Here's how the part is built. I have some questions about the finished solid (model axes, mm). Give positions to 0.01 mm unless a question says otherwise; leave off trailing zeros. Write each loop counter-clockwise with the first axis right and the second up, starting at its lowest first coordinate (ties: lowest second). Pieces come first, ordered by that corner, then holes. Notation, with made-up numbers: (77.5, -6.5) -> (95.5, -6.5) arc R24 ccw to (95.5, 20.5) -> close; hole circle Ø7 at (-26, -38.5). An arc over 180 degrees is marked (long way). Use CSV: the item, a comma, the result in double quotes. Start each with the question number.
(1) Suppose I cut it at D-D on y = -4.5. List the corners of the cut face in (x, z) for me, plus the area to 3 significant figures.
(2) I need wall thicknesses on L1, parallel to Y at x = -33, z = -0.5; L2, parallel to Z at x = 30, y = -0.25; L3, parallel to Z at x = 34.5, y = -6.5. Which ranges of each line are inside material? Lowest first, please. Write a range as [from, to].
(3) Suppose I cut it at B-B on z = 19.05. List the corners of the cut face in (x, y) for me (3 decimals).
(4) For pin 1 Ø4 at (x, y) = (39.5, 7) entering from -Z; pin 2 Ø6 at (x, y) = (-17.5, 6) entering from +Z; pin 3 Ø4 at (x, y) = (-48.5, -4) entering from -Z, each with a flat end and sliding along its axis, tell me the tip position at first contact or that it passes through.
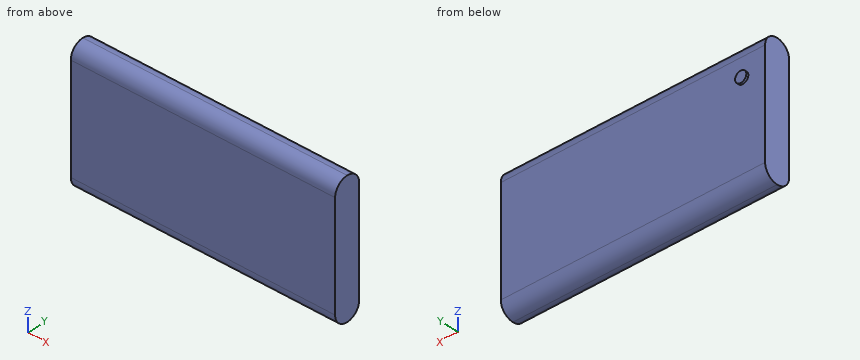
from build123d import *

# Parameters (mm, degrees)
SKETCH1_W           = 150
SKETCH1_H           = 75
BOSS_EXTRUDE1_DEPTH = 7.5
FILLET1_R           = 7.5
SKETCH2_R           = 3.175
BOSS_EXTRUDE2_DEPTH = 1.27


with BuildPart() as part:
    # Sketch1 → Boss-Extrude1 (new, symmetric)
    with BuildSketch(Plane(origin=(0, 0, 0), x_dir=(1, 0, 0), z_dir=(0, 1, 0))):
        Rectangle(SKETCH1_W, SKETCH1_H)
    extrude(amount=BOSS_EXTRUDE1_DEPTH, both=True)

    # Fillet1
    fillet1_edges = [part.edges().sort_by_distance(p)[0] for p in [
        (0, -7.5, -37.5),
        (0, 7.5, -37.5),
        (0, -7.5, 37.5),
        (0, 7.5, 37.5),
    ]]
    fillet(fillet1_edges, radius=FILLET1_R - 0.0001)  # a hair under: the kernel refuses the full size

    # Sketch2 → Boss-Extrude2 (add)
    with BuildSketch(Plane(origin=(0, 7.5, 0), x_dir=(1, 0, 0), z_dir=(0, 1, 0))):
        with Locations(Location((-62.3, -19.05, 0), (0, 0, 90))):
            Circle(SKETCH2_R)
    extrude(amount=BOSS_EXTRUDE2_DEPTH)


solid = part.part
Geometry says:
1,outline,"(-75, -36) -> (75, -36) -> (75, 36) -> (-75, 36) -> close"
1,area,"10,800 mm²"
2,L1,"[-7.5, 7.5]"
2,L2,"[-37.5, 37.5]"
2,L3,"[-33.74, 33.74]"
3,outline,"(-75, -7.5) -> (75, -7.5) -> (75, 7.5) -> (-59.125, 7.5) -> (-59.125, 8.77) -> (-65.475, 8.77) -> (-65.475, 7.5) -> (-75, 7.5) -> close"
4,pin 1,"z = -35.59"
4,pin 2,"z = 36.87"
4,pin 3,"z = -37.23"
